Could you check a few things on this model? Use its own coordinates, in mm. Coordinates: 2 decimals unless noted, no trailing zeros. Loops run counter-clockwise (first coordinate to the right, second up) from the corner with the lowest first, then second, coordinate; pieces in that order, holes last. Notation, with made-up numbers: (-9, 68.25) -> (50, 68.25) arc R37 ccw to (50, 107.25) -> close; hole circle Ø8 at (39, 86). An arc over 180 degrees is marked (long way). One line per question, with ' | ' between items.
```python
from build123d import *

# Parameters (mm, degrees)
SCHIZZO1_R                   = 55
SCHIZZO1_R_2                 = 52
ESTRUSIONE_ESTRUSIONE1_DEPTH = 5
SMUSSO1_SIZE                 = 0.2


with BuildPart() as part:
    # Schizzo1 → Estrusione-Estrusione1 (new body)
    with BuildSketch(Plane.XY):
        Circle(SCHIZZO1_R)
        Circle(SCHIZZO1_R_2, mode=Mode.SUBTRACT)
    extrude(amount=ESTRUSIONE_ESTRUSIONE1_DEPTH)

    # Smusso1
    smusso1_edges = [part.edges().sort_by_distance(p)[0] for p in [
        (-55, 0, 0),
        (-55, 0, 5),
        (-52, 0, 0),
        (-52, 0, 5),
    ]]
    chamfer(smusso1_edges, length=SMUSSO1_SIZE)


solid = part.part
```
Q1. We'd pull the mould along Y, two halves only. Please class faces 1 (the face through (-11.923, -53.692, 2.468)), 2 (the face through (-41.265, -31.641, 2.468)), 3 (the face through (48.5, -20, 0)): released by +Y, released by -Y, zero draft, split by the parting line, or undercut.
Values follow:
face 1: split by the parting line | face 2: undercut | face 3: zero draft
Q2. Imagine slicing it at A-A on y = 0. Write out the boundary of the cut face in (x, z).
Values follow:
outline: (-55, 0.2) -> (-54.8, 0) -> (-52.2, 0) -> (-52, 0.2) -> (-52, 4.8) -> (-52.2, 5) -> (-54.8, 5) -> (-55, 4.8) -> close; (52, 0.2) -> (52.2, 0) -> (54.8, 0) -> (55, 0.2) -> (55, 4.8) -> (54.8, 5) -> (52.2, 5) -> (52, 4.8) -> close
Q3. For pin 1 (3 mm diameter, centred on x = -18, z = 0.5, fed in from +Y); pin 2 (3 mm diameter, centred on y = 17.5, z = 3, fed in from -X); pin 3 (1.5 mm diameter, centred on x = 25.5, z = 2, fed in from +Y), each with a flat end and sliding along its axis, tell me the tip position at first contact or that it passes through.
Values follow:
pin 1: stops at y = 52.47 | pin 2: stops at x = -52.62 | pin 3: stops at y = 49.12
Q4. Please list where these lines run through material, in increasing order: L1, parallel to Y at x = 0, z = 3.75; L2, parallel to Y at x = 40.5, z = 0.4; L3, parallel to X at y = 19, z = 0.85. Write a range as [from, to].
Values follow:
L1: y = [-55, -52], [52, 55] | L2: y = [-37.21, -32.62], [32.62, 37.21] | L3: x = [-51.61, -48.4], [48.4, 51.61]
Q5. Imagine slicing it at C-C on z = 3.3. Write out the boundary of the cut face in (x, y).
Values follow:
outline: circle Ø110 at (0, 0); hole circle Ø104 at (0, 0)
